Build history of the part. All positions in model axes, mm. Face numbers are marked on the shaded views. A direction names the side the tool comes from. Coordinates: 2 decimals unless noted, no trailing zeros. Order: outer loops, then holes, each group sorted by start corner. A loop starts at its lowest first (then second) coordinate and runs counter-clockwise, first axis right, second up. Notation, with made-up numbers: M 44.5,28.5 L 62.5,28.5 A7 cw 62.5,41.5 Z; hole C -23.5,-0.5 d7. An arc over 180 degrees is marked long. Use a Markdown table: item, result. Add a question column.
Autodesk Inventor part; units mm, degrees
ref_plane "YZ Plane" through (0, 0, 0) normal (1, 0, 0) x (0, 1, 0)
ref_plane "XZ Plane" through (0, 0, 0) normal (0, 1, 0) x (-1, 0, 0)
ref_plane "XY Plane" through (0, 0, 0) normal (0, 0, 1) x (1, 0, 0)
sketch "Эскиз1" plane through (0, 0, 0) normal (0, 1, 0) x (-1, 0, 0)
  circle A0 centre (0, 0) radius 12.5
  circle A1 centre (0, 0) radius 18.5
  dimension "d0" = 25
  dimension "d1" = 37
extrude "Выдавливание1" add sketch "Эскиз1" along normal mid plane 7
sketch "Эскиз2" plane through (0, 3.5, 0) normal (0, 1, 0) x (1, 0, 0)
  circle A0 centre (0, 0) radius 14.2
  circle A1 centre (0, 0) radius 16.8
  circle A2 centre (0, 0) radius 12.5
  dimension "d4" = 2.6
  dimension "d5" = 1.7
extrude "Выдавливание2" cut sketch "Эскиз2" against normal blind 0.5 contours A1
chamfer "Фаска2" distance 0.4 angle 45 4 edges at (18.5, -3.5, 0) (18.5, 3.5, 0) (12.5, -3.5, 0) (12.5, 3.5, 0)
sketch "Эскиз3" plane through (0, -3.5, 0) normal (0, -1, 0) x (1, 0, 0)
  circle A0 centre (0, 0) radius 16.8
  circle A1 centre (0, 0) radius 14.2
extrude "Выдавливание3" cut sketch "Эскиз3" against normal blind 0.5
chamfer "Фаска1" distance 0.25 angle 45 4 edges at (-16.8, 3.5, 0) (-14.2, 3.5, 0) (-16.8, -3.5, 0) (-14.2, -3.5, 0)
properties part number "bearing 37x25x7"
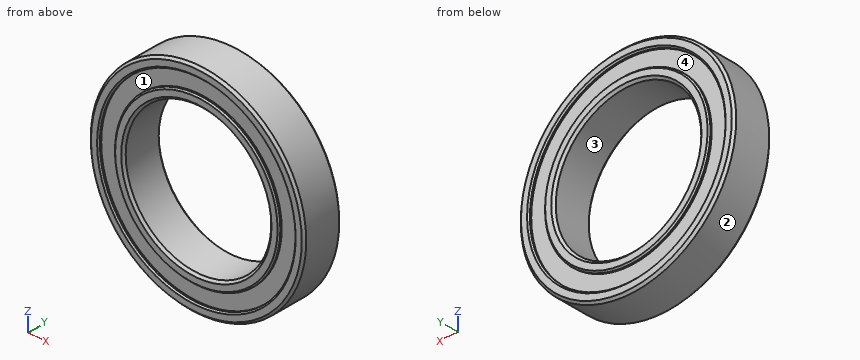
(1) Which spindle directions (+Z, -Z, +X, -X, +Y, -Y) get a long thin tool onto all of the face, cutting with end or side? Do the marked faces 3 and 4. Say none if no direction does.
(2) Slice it at A-A on y = 1. Give the cut face in (x, z).
(3) Drop flat-ended pins along their axis: P1, Ø1, axis at x = 2.5, z = -10.5, coming from the +Y side; P2, Ø2, axis at y = 0.5, z = 8, coming from the -X side; P3, Ø2, axis at x = -11, y = 1.5, coming from the -Z side; P4, Ø2, axis at x = -3, y = -1.5, coming from the -Z side. Give the stop position or say it passes through.
(4) Drill centre lines: line 1 along Z through (x, y) = (0, -3.05); line 2 along Z through (x, y) = (0, 3.15); line 3 along Z through (x, y) = (0, -0.5). Where is each one in solid material? Low to high. Write a range as from..to.
(5) Mould opens along X. For the marked faces 1 and 2 say: released by +X, released by -X, zero draft, split by the parting line, or undercut.
Solutions:
| question | item | result |
|---|---|---|
| 1 | face 3 | +Y, -Y |
| 1 | face 4 | +Y |
| 2 | outline | C 0,0 d37; hole C 0,0 d25 |
| 3 | P1 | through |
| 3 | P2 | x = -17.12 |
| 3 | P3 | z = -15.56 |
| 3 | P4 | z = -18.39 |
| 4 | line 1 | -18.5..-16.8, -14.2..-12.5, 12.5..14.2, 16.8..18.5 |
| 4 | line 2 | -18.45..-16.8, -14.2..-12.55, 12.55..14.2, 16.8..18.45 |
| 4 | line 3 | -18.5..-12.5, 12.5..18.5 |
| 5 | face 1 | undercut |
| 5 | face 2 | split by the parting line |
